from build123d import *

# Parameters (mm, degrees)
SKETCH1_R           = 2.286
BOSS_EXTRUDE1_DEPTH = 7.3025
SKETCH2_R           = 2.38252
BOSS_EXTRUDE2_DEPTH = 4.762246
SKETCH3_R           = 3.175
BOSS_EXTRUDE3_DEPTH = 3.175
SKETCH4_R           = 3.175
BOSS_EXTRUDE4_DEPTH = 3.175
THREAD2_PITCH       = 1.27
SKETCH11_R          = 6.35
BOSS_EXTRUDE5_DEPTH = 3.81


with BuildPart() as part:
    # Sketch1 → Boss-Extrude1 (new body)
    with BuildSketch(Plane(origin=(0, 0, 0), x_dir=(1, 0, 0), z_dir=(0, 1, 0))):
        with Locations(Location((0, 0, 0), (0, 0, 90))):
            Circle(SKETCH1_R)
    extrude(amount=BOSS_EXTRUDE1_DEPTH)

    # Sketch2 → Boss-Extrude2 (add)
    with BuildSketch(Plane(origin=(0, 0, 0), x_dir=(-1, 0, 0), z_dir=(0, -1, 0))):
        with Locations(Location((0, 0, 0), (0, 0, 90))):
            Circle(SKETCH2_R)
    extrude(amount=BOSS_EXTRUDE2_DEPTH)

    # Sketch3 → Boss-Extrude3 (add)
    with BuildSketch(Plane(origin=(0, -4.762246, 0), x_dir=(-1, 0, 0), z_dir=(0, -1, 0))):
        with Locations(Location((0, 0, 0), (0, 0, 90))):
            Circle(SKETCH3_R)
    extrude(amount=BOSS_EXTRUDE3_DEPTH)

    # Sketch4 → Boss-Extrude4 (add)
    with BuildSketch(Plane(origin=(0, -7.937246, 0), x_dir=(-1, 0, 0), z_dir=(0, -1, 0))):
        with Locations(Location((0, 0, 0), (0, 0, 90))):
            Circle(SKETCH4_R)
    extrude(amount=BOSS_EXTRUDE4_DEPTH)

    # Thread2: the profile of Thread Profile3 profile screwed along a right-hand helix of 3.75 turns, 8 arcs to a turn; built about Z, then put on its axis
    thread2_z = Axis((0, 0, 0), (0, 0, 1))
    thread2_corners = [(3.1753, 0, -0.000173205), (3.1753, 0, 1.111423202), (2.487592339, 0, 0.714374998), (2.487592339, 0, 0.396874998)]
    with BuildLine(mode=Mode.PRIVATE) as thread2_profile:
        Line(thread2_corners[0], thread2_corners[1])
        Line(thread2_corners[1], thread2_corners[2])
        Line(thread2_corners[2], thread2_corners[3])
        Line(thread2_corners[3], thread2_corners[0])
    thread2_cap = Face(thread2_profile.wire())
    thread2_turn_angles = [0, 22.5, 45, 67.5, 90, 112.5, 135, 157.5, 180, 202.5, 225, 247.5, 270, 292.5, 315, 337.5, 360]
    thread2_turn_weights = [1, 0.9238795325112867, 1, 0.9238795325112867, 1, 0.9238795325112867, 1, 0.9238795325112867, 1, 0.9238795325112867, 1, 0.9238795325112867, 1, 0.9238795325112867, 1, 0.9238795325112867, 1]
    thread2_turn_rails = [Edge.make_bspline([Vector(p[0], p[1], 0).rotate(thread2_z, thread2_turn_angles[k]) / thread2_turn_weights[k] + Vector(0, 0, p[2] + THREAD2_PITCH * thread2_turn_angles[k] / 360) for k in range(17)], [0, 0, 0, 1, 1, 2, 2, 3, 3, 4, 4, 5, 5, 6, 6, 7, 7, 8, 8, 8], 2, thread2_turn_weights) for p in thread2_corners]
    thread2_turn_sides = [Face.make_surface_from_curves(thread2_turn_rails[p[0]], thread2_turn_rails[p[1]]) for p in [(0, 1), (1, 2), (2, 3), (3, 0)]]
    thread2_last_angles = [1080, 1102.5, 1125, 1147.5, 1170, 1192.5, 1215, 1237.5, 1260, 1282.5, 1305, 1327.5, 1350]
    thread2_last_weights = [1, 0.9238795325112867, 1, 0.9238795325112867, 1, 0.9238795325112867, 1, 0.9238795325112867, 1, 0.9238795325112867, 1, 0.9238795325112883, 1]
    thread2_last_rails = [Edge.make_bspline([Vector(p[0], p[1], 0).rotate(thread2_z, thread2_last_angles[k]) / thread2_last_weights[k] + Vector(0, 0, p[2] + THREAD2_PITCH * thread2_last_angles[k] / 360) for k in range(13)], [0, 0, 0, 1, 1, 2, 2, 3, 3, 4, 4, 5, 5, 6, 6, 6], 2, thread2_last_weights) for p in thread2_corners]
    thread2_last_sides = [Face.make_surface_from_curves(thread2_last_rails[p[0]], thread2_last_rails[p[1]]) for p in [(0, 1), (1, 2), (2, 3), (3, 0)]]
    thread2 = Plane(origin=(0, -9.524746, 0), x_dir=(1, 0, 0), z_dir=(0, 1, 0)) * Solid(Shell([*[p.moved(Location((0, 0, THREAD2_PITCH * i))) for i in range(3) for p in thread2_turn_sides], *thread2_last_sides, thread2_cap, thread2_cap.rotate(thread2_z, 1350).moved(Location((0, 0, THREAD2_PITCH * 1350 / 360)))]))
    add(thread2, mode=Mode.SUBTRACT)

    # Sketch11 → Boss-Extrude5 (add)
    with BuildSketch(Plane(origin=(0, -11.112246, 0), x_dir=(-1, 0, 0), z_dir=(0, -1, 0))):
        with Locations(Location((0, 0, 0), (0, 0, 270))):
            Circle(SKETCH11_R)
    extrude(amount=BOSS_EXTRUDE5_DEPTH)


solid = part.part
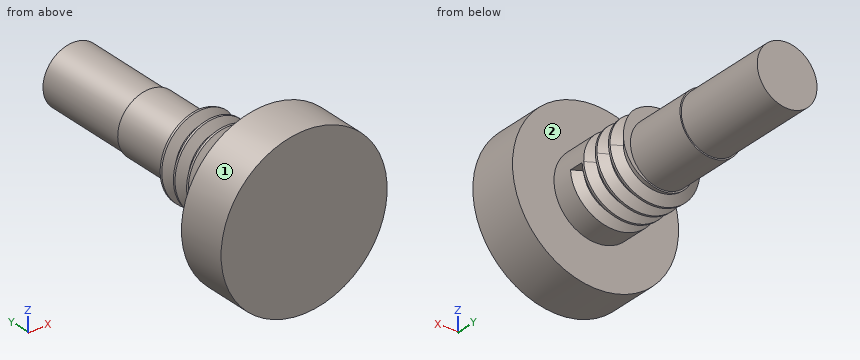
For this review, take the finished solid that the model builds, in its own axes (mm). Face numbers are marked on the shaded views. A direction names the side the tool comes from. Coordinates: 2 decimals unless noted, no trailing zeros. Order: outer loops, then holes, each group sorted by start corner. A loop starts at its lowest first (then second) coordinate and runs counter-clockwise, first axis right, second up. Notation, with made-up numbers: (-26, 34.25) - (26, 34.25) arc R22 cw to (26, 45.25) - close; hole circle Ø11 at (18.5, -4.5). An arc over 180 degrees is marked (long way). Use one line per item in the form item = value.
Q1. For P1, Ø2, axis at y = -11, z = -2, coming from the +X side; P2, Ø5, axis at x = 2.5, y = 5, coming from the -Z side; P3, Ø5, axis at y = -4, z = -1, coming from the +X side (3 decimals), all flat-tipped, find the tip position at first contact; note any pin that passes through.
Checked values:
P1 = 6.27
P2 = -2.29
P3 = 3.175
Q2. Consider section B-B (z = 4). Give the boundary of the cut face in (x, y), then the cut area to 3 significant figures.
Checked values:
outline = (-4.93, -14.92) - (4.93, -14.92) - (4.93, -11.11) - (-4.93, -11.11) - close
area = 37.6 mm2
Q3. Consider section D-D (z = -2.75). Give the number of separate pieces and of enclosed holes in the cut face, then the cut area to 3 significant figures.
Checked values:
separate_pieces = 4
enclosed_holes = 0
area = 54.8 mm2
Q4. Consider section C-C (x = -4.75). Give the boundary of the cut face in (y, z).
Checked values:
outline = (-14.92, -4.21) - (-11.11, -4.21) - (-11.11, 4.21) - (-14.92, 4.21) - close
Q5. For the marked faces 1 and 2, list the 3-axis set-ups (+Z, -Z, +X, -X, +Y, -Y) from which the entire face can be reached by the end or side of a thin tool; tool diameter is ignored.
Checked values:
face_1 = +Y, -Y
face_2 = +Y
Q6. For probe 1 along Y at (x, z) = (-1.5, 2.75); probe 2 along Y at (x, z) = (2, 4.25); probe 3 along X at (y, z) = (-10.5, 0.25), list the stretches that pass through material, from the lowest coordinate up. Write a range as from..to.
Checked values:
probe_1 = -14.92..-8.65, -7.59..-7.38, -6.32..-6.11, -5.05..-4.84
probe_2 = -14.92..-11.11
probe_3 = -3.17..3.17
Q7. Consider section A-A (y = 1.5). Give the boundary of the cut face in (x, z), then the cut area to 3 significant figures.
Checked values:
outline = circle Ø4.57 at (0, 0)
area = 16.4 mm2
